Model file for the job. Use its own axes, mm. A direction names the side the tool comes from. Coordinates: 2 decimals unless noted, no trailing zeros. Write each loop counter-clockwise with the first axis right and the second up, starting at its lowest first coordinate (ties: lowest second). Pieces come first, ordered by that corner, then holes. Notation, with made-up numbers: M 44.25,-14.75 L 87.25,-14.75 A15 cw 87.25,1.25 Z; hole C 81,-18 d9. An arc over 180 degrees is marked long. Put each result on its own line as item: value. Start each with the question number.
Q1. Pull direction Y, two halves, no side cores. Call faces 1 (the flat face through (0, -587.5, 0)), 2 (the cylindrical face through (11.41, -300.08, -14.88)), 3 (the flat face through (13, 0, -8)): pulls with the +Y half, pulls with the -Y half, needs draft (parallel to the pull), parting line crosses it, or undercut.
Q2. Cut at C-C (y = -513). Write the cut outline in (x, z).
Q3. Cut at A-A (x = 8.5). Write the cut outline in (y, z).
Q4. Which spindle directions (+Z, -Z, +X, -X, +Y, -Y) get a long thin tool onto all of the face, cutting with end or side? Do faces 4 (the cylindrical face through (-11.41, 6.16, -14.88)), 5 (the flat face through (-13, -4.5, -8)). Say none if no direction does.
Q5. Drill centre lines: line 1 along Y through (x, z) = (17.5, -2); line 2 along X through (y, z) = (-172, 0); line 3 along Z through (x, y) = (-1, -484). Where is each one in solid material? Low to high.
Q6. Cut at B-B (z = -6.5). Write the cut outline in (x, y).
Q7. Drop flat-ended pins along their axis: pin 1 (8 mm diameter, centred on y = -438.5, z = 0, fed in from -X); pin 2 (2 mm diameter, centred on y = -320.5, z = -5.5, fed in from -X); pin 3 (1 mm diameter, centred on x = 4.5, y = -365, fed in from -Z). Give the stop position or say it passes through.
```python
from build123d import *

# Parameters (mm, degrees)
SKETCH1_R           = 18.75
BOSS_EXTRUDE1_DEPTH = 12.5
SKETCH2_R           = 15
BOSS_EXTRUDE2_DEPTH = 4.5
BOSS_EXTRUDE3_START = 583
SKETCH3_R           = 18.75
BOSS_EXTRUDE3_DEPTH = 583


with BuildPart() as part:
    # Sketch1 → Boss-Extrude1 (new body)
    with BuildSketch(Plane(origin=(0, 0, 0), x_dir=(1, 0, 0), z_dir=(0, 1, 0))):
        with Locations(Location((0, 0, 0), (0, 0, 270))):
            Circle(SKETCH1_R)
    extrude(amount=BOSS_EXTRUDE1_DEPTH)

    # Sketch2 → Boss-Extrude2 (add)
    with BuildSketch(Plane.XZ):
        with Locations(Location((0, 0, 0), (0, 0, 270))):
            Circle(SKETCH2_R)
    extrude(amount=BOSS_EXTRUDE2_DEPTH)

    # Sketch3 → Boss-Extrude3 (add)
    with BuildSketch(Plane.XZ.offset(4.5).offset(BOSS_EXTRUDE3_START)):
        with Locations(Location((0, 0, 0), (0, 0, 90))):
            Circle(SKETCH3_R)
    extrude(amount=-BOSS_EXTRUDE3_DEPTH)


solid = part.part
```
Computed values:
1. face 1: pulls with the -Y half
1. face 2: needs draft
1. face 3: undercut
2. outline: C 0,0 d37.5
3. outline: M -587.5,-16.71 L -4.5,-16.71 L -4.5,-12.36 L 0,-12.36 L 0,-16.71 L 12.5,-16.71 L 12.5,16.71 L 0,16.71 L 0,12.36 L -4.5,12.36 L -4.5,16.71 L -587.5,16.71 Z
4. face 4: +Y, -Y
4. face 5: none
5. line 1: -587.5 to -4.5, 0 to 12.5
5. line 2: -18.75 to 18.75
5. line 3: -18.72 to 18.72
6. outline: M -17.59,-587.5 L 17.59,-587.5 L 17.59,-4.5 L 13.52,-4.5 L 13.52,0 L 17.59,0 L 17.59,12.5 L -17.59,12.5 L -17.59,0 L -13.52,0 L -13.52,-4.5 L -17.59,-4.5 Z
7. pin 1: x = -18.75
7. pin 2: x = -18.2
7. pin 3: z = -18.32
